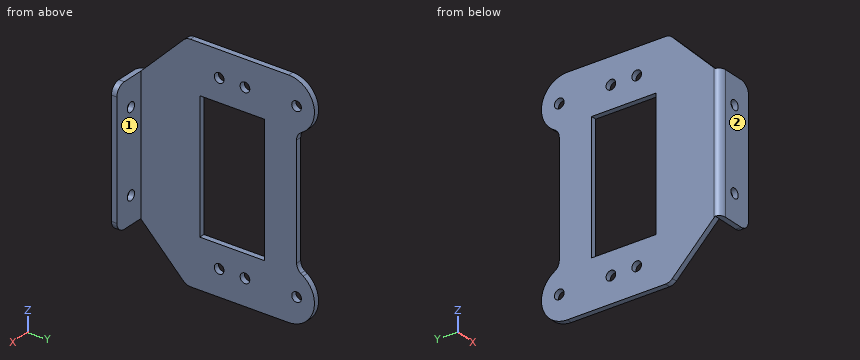
Autodesk Inventor part; units mm, degrees
ref_plane "YZ Plane" through (0, 0, 0) normal (1, 0, 0) x (0, 1, 0)
ref_plane "XZ Plane" through (0, 0, 0) normal (0, 1, 0) x (-1, 0, 0)
ref_plane "XY Plane" through (0, 0, 0) normal (0, 0, 1) x (1, 0, 0)
sketch "Sketch1" plane through (0, 0, 0) normal (0, 1, 0) x (-1, 0, 0)
  line L0 (0, 12.5) -> (0, -12.5) construction
  line L1 (-1.5, 12.5) -> (-1.5, -12.5)
  line L2 (1.5, -12.5) -> (1.5, 12.5)
  arc A0 (1.5, 12.5) -> (-1.5, 12.5) centre (0, 12.5) ccw
  arc A1 (-1.5, -12.5) -> (1.5, -12.5) centre (0, -12.5) ccw
  circle A2 centre (0, -12.5) radius 1.5
  circle A3 centre (0, 12.5) radius 1.5
  line L3 (-5.7579, 20.8654) -> (5.7579, 20.8654)
  line L4 (5.7579, 20.8654) -> (5.7579, -20.8654)
  line L5 (5.7579, -20.8654) -> (-5.7579, -20.8654)
  line L6 (-5.7579, -20.8654) -> (-5.7579, 20.8654)
  line L7 (-5.7579, 20.8654) -> (5.7579, -20.8654) construction
  line L8 (5.7579, 20.8654) -> (-5.7579, -20.8654) construction
  point P0 (0, 0)
  dimension "d0" = 12.5
  dimension "d1" = 3
  dimension "d2" = 3
  dimension "d3" = 3
extrude "Extrusion1" add sketch "Sketch1" along normal blind 1.7 contours A3 L2 A2 L1 | L3 L4 L5 L6
sketch "Sketch2" plane through (-5.7579, 0, -20.8654) normal (-1, 0, 0) x (0, 0, 1)
  line L0 (40.8654, 20) -> (0.8654, 20)
  line L1 (0.8654, 20) -> (0.8654, 40)
  line L2 (0.8654, 40) -> (40.8654, 40)
  line L3 (40.8654, 40) -> (40.8654, 20)
  line L4 (40.8654, 20) -> (0.8654, 40) construction
  line L5 (0.8654, 20) -> (40.8654, 40) construction
  line L6 (41.7309, 0) -> (0, 0)
  circle A0 centre (47.8654, 50) radius 1.5
  circle A1 centre (-6.1346, 50) radius 1.5
  line L7 (0, 1.7) -> (41.7309, 1.7)
  line L8 (41.7309, 1.7) -> (55.873, 15.8421)
  line L9 (41.7309, 1.7) -> (61.7309, 1.7) construction
  line L10 (55.873, 15.8421) -> (55.873, 55.8421)
  line L11 (55.873, 15.8421) -> (95.873, 15.8421) construction
  line L12 (0, 1.7) -> (-14.1421, 15.8421)
  line L13 (0, 1.7) -> (20, 1.7) construction
  line L14 (-14.1421, 15.8421) -> (-14.1421, 55.8421)
  line L15 (-14.1421, 55.8421) -> (55.873, 55.8421)
  point P0 (20.8654, 0)
  point P1 (20.8654, 30)
  dimension "d6" = 40
  dimension "d7" = 20
  dimension "d8" = 30
  dimension "d9" = 3
  dimension "d10" = 3
  dimension "d11" = 50
  dimension "d12" = 50
  dimension "d13" = 54
  dimension "d14" = 27
  dimension "d15" = 20
  dimension "d16" = 45
  dimension "d17" = 40
  dimension "d18" = 90
  dimension "d19" = 20
  dimension "d20" = 135
  dimension "d21" = 40
extrude "Extrusion2" add sketch "Sketch2" against normal blind 1.7
sketch "Sketch3" plane through (-4.0579, 0, -20.8654) normal (1, 0, 0) x (0, 0, -1)
  line L0 (-55.873, 55.8421) -> (14.1421, 55.8421)
  line L1 (-43.8654, 55.8421) -> (-39.8654, 50)
  line L2 (-39.8654, 50) -> (-1.8654, 50)
  line L3 (-1.8654, 50) -> (2.1346, 55.8421)
  line L4 (-40.8654, 40) -> (-0.8654, 40)
  circle A0 centre (-47.8654, 50) radius 1.5
  circle A1 centre (6.1346, 50) radius 1.5
  line L5 (14.1421, 55.8421) -> (-55.873, 55.8421)
  line L6 (-43.8654, 55.8421) -> (2.1346, 55.8421)
  point P0 (-20.8654, 0)
  point P1 (2.1346, 55.8421)
  dimension "d24" = 10
  dimension "d25" = 4
  dimension "d26" = 4
  dimension "d27" = 4
  dimension "d28" = 4
extrude "Extrusion3" cut sketch "Sketch3" against normal blind 10 contours L0 L3 L2 L1
fillet "Fillet1" radius 8 4 edges at (-4.9079, 55.8421, 35.0076) (-4.9079, 55.8421, 23) (-4.9079, 55.8421, -23) (-4.9079, 55.8421, -35.0076)
fillet "Fillet2" radius 3 2 edges at (-4.9079, 50, -19) (-4.9079, 50, 19)
fillet "Fillet3" radius 3 4 edges at (-4.9079, 15.8421, -35.0076) (5.7579, 0.85, -20.8654) (5.7579, 0.85, 20.8654) (-4.9079, 15.8421, 35.0076)
fillet "Fillet4" radius 2 1 edges at (-5.7579, 0, 0)
sketch "Sketch4" plane through (-4.0579, 0, -20.8654) normal (1, 0, 0) x (0, 0, -1)
  line L0 (-47.8654, 34) -> (6.1346, 34)
  line L1 (6.1346, 34) -> (6.1346, 26)
  line L2 (6.1346, 26) -> (-47.8654, 26)
  line L3 (-47.8654, 26) -> (-47.8654, 34)
  line L4 (-0.8654, 20) -> (-40.8654, 20)
  line L5 (-0.8654, 40) -> (-0.8654, 20)
  circle A0 centre (-47.8654, 34) radius 1.5
  circle A1 centre (-47.8654, 26) radius 1.5
  circle A2 centre (6.1346, 34) radius 1.5
  circle A3 centre (6.1346, 26) radius 1.5
  point P0 (-20.8654, 0)
  dimension "d35" = 54
  dimension "d36" = 8
  dimension "d37" = 6
  dimension "d38" = 7
  dimension "d39" = 3
  dimension "d40" = 3
  dimension "d41" = 3
  dimension "d42" = 3
extrude "Extrusion4" cut sketch "Sketch4" against normal blind 10 contours L3 A0 L0 | L0 A0 L3 | A1 L2 L3 | L3 L2 A1 | A2 L1 L0 | L0 L1 A2 | A3 L1 L2 | L2 L1 A3
properties part number "servo mount"
The listing builds one solid part. Answer for the finished solid, in the listing's coordinates (mm). Face numbers are marked on the shaded views. A direction names the side the tool comes from. Give positions to 0.01 mm unless a question says otherwise; leave off trailing zeros. Write each loop counter-clockwise with the first axis right and the second up, starting at its lowest first coordinate (ties: lowest second). Pieces come first, ordered by that corner, then holes. Notation, with made-up numbers: M 58.5,13 L 117.5,13 A11 cw 117.5,28 Z; hole C 23.25,-25.5 d7. An arc over 180 degrees is marked long. Write each question's results on one line, items separated by ' | '.
Q1. Section B-B, the plane x = 0 is taken. Write down the section's boundary in (y, z).
Output values:
outline: M 0,-20.87 L 1.7,-20.87 L 1.7,-14 L 0,-14 Z; M 0,-11 L 1.7,-11 L 1.7,11 L 0,11 Z; M 0,14 L 1.7,14 L 1.7,20.87 L 0,20.87 Z
Q2. Section D-D, the plane z = 27 is taken. Count the separate pieces of the cut face and the enclosed holes in it, then the cut area to 3 significant figures.
Output values:
separate pieces: 4 | enclosed holes: 0 | area: 65.8 mm2
Q3. Flat-ended cylindrical pins translate along their axes: P1, Ø0.5, axis at x = -4.5, z = -1, coming from the +Y side; P2, Ø1.4, axis at x = -5, z = 7, coming from the -Y side; P3, Ø1.4, axis at x = -3.5, y = 0.5, coming from the +Z side. Find the tip coordinate at first contact, or state that the pin passes through.
Output values:
P1: y = 50 | P2: y = 0.07 | P3: z = 20.87
Q4. Consider L1, parallel to Z at x = -4.65, y = 26; L2, parallel to Z at x = 0, y = 1.3; L3, parallel to Y at x = -4.65, z = 27. Determine where each line is inside the solid, lowest interval first. Write a range as from..to.
Output values:
L1: -35.01..-28.5, -25.5..-20, 20..25.5, 28.5..35.01 | L2: -20.87..-14, -11..11, 14..20.87 | L3: 7.83..24.5, 27.5..32.5, 35.5..48.5, 51.5..55.54
Q5. Section A-A, the plane z = -12.5 is taken. Write down the section's boundary in (x, y), then the cut area to 3 significant figures.
Output values:
outline: M -5.76,2 A2 ccw -3.76,0 L -1.5,0 L -1.5,1.7 L -4.06,1.7 L -4.06,20 L -5.76,20 Z; M -5.76,40 L -4.06,40 L -4.06,50 L -5.76,50 Z; M 1.5,0 L 5.76,0 L 5.76,1.7 L 1.5,1.7 Z | area: 61.7 mm2
Q6. Section C-C, the plane y = 34 is taken. Write down the section's boundary in (x, z), then the cut area to 3 significant figures.
Output values:
outline: M -5.76,-35.01 L -4.06,-35.01 L -4.06,-28.5 L -5.76,-28.5 Z; M -5.76,-25.5 L -4.06,-25.5 L -4.06,-20 L -5.76,-20 Z; M -5.76,20 L -4.06,20 L -4.06,25.5 L -5.76,25.5 Z; M -5.76,28.5 L -4.06,28.5 L -4.06,35.01 L -5.76,35.01 Z | area: 40.8 mm2
Q7. A tool of negligible diameter and unlimited length cuts with its end or side. For the marked faces 1 and 2, from which of +Z, -Z, +X, -X, +Y, -Y can it reach the whole face along a straight path? Write none if from no direction.
Output values:
face 1: +Z, -Z, +X, +Y | face 2: +Z, -Z, +X, -X, -Y
